```python
from build123d import *

# Parameters (mm, degrees)
ESQUISSE5_W                  = 10
ESQUISSE5_H                  = 23
ESQUISSE5_W_2                = 260
ESQUISSE5_H_2                = 10
ESQUISSE5_W_3                = 9.9238066
BOSS_EXTRU_4_DEPTH           = 81
ENL_V_MAT_EXTRU_2_DEPTH      = 2
ENL_V_MAT_EXTRU_2_DEPTH_BACK = 227


with BuildPart() as part:
    # Esquisse5 → Boss.-Extru.4 (new body)
    with BuildSketch(Plane(origin=(0, 0, 0), x_dir=(1, 0, 0), z_dir=(0, 1, 0))):
        Polygon((0, 32.998552378), (0, 23), (10, 23), (250.0761934, 23), (260, 23), (260, 32.998552378), align=None)
        with Locations((5, 11.5)):
            Rectangle(ESQUISSE5_W, ESQUISSE5_H)
        with Locations((130, -5)):
            Rectangle(ESQUISSE5_W_2, ESQUISSE5_H_2)
        with Locations((255.0380967, 11.5)):
            Rectangle(ESQUISSE5_W_3, ESQUISSE5_H)
    extrude(amount=BOSS_EXTRU_4_DEPTH)

    # Esquisse7 → Enlèv. mat.-Extru.2 (cut, two sides: drawn at the far end of the back side and taken through both)
    with BuildSketch(Plane(origin=(0, 0, -32.998552378), x_dir=(-1, 0, 0), z_dir=(0, 0, -1)).offset(-ENL_V_MAT_EXTRU_2_DEPTH_BACK)):
        Polygon((0, 0), (0, 81), (-39.230090492, 0), align=None)
    extrude(amount=ENL_V_MAT_EXTRU_2_DEPTH + ENL_V_MAT_EXTRU_2_DEPTH_BACK, mode=Mode.SUBTRACT)


solid = part.part
```
Part model, mm, in its own coordinate system. A direction names the side the tool comes from. Give positions to 0.01 mm unless a question says otherwise; leave off trailing zeros. Order: outer loops, then holes, each group sorted by start corner. A loop starts at its lowest first (then second) coordinate and runs counter-clockwise, first axis right, second up. Notation, with made-up numbers: (-16.5, 16.5) - (37.5, 16.5) arc R16 ccw to (37.5, 42.5) - close; hole circle Ø10 at (47, 68.25). An arc over 180 degrees is marked (long way). Use one line per item in the form item = value.
Item 1: Probe probe 1 along Z at (x, y) = (59, 72.5); probe 2 along X at (y, z) = (43, -14); probe 3 along X at (y, z) = (76, -8). List the from-to ranges inside material, lowest first. Write a range as from..to.
Solution:
probe_1 = -33..-23, 0..10
probe_2 = 250.08..260
probe_3 = 2.42..10, 250.08..260
Item 2: Two-plate mould, pull along X, no slides. Class faces 3 (the face through (10, 71, -11)), 4 (the face through (260, 40, -11)), 5 (the face through (148, 0, -26)): released by +X, released by -X, zero draft, split by the parting line, or undercut.
Solution:
face_3 = undercut
face_4 = released by +X
face_5 = zero draft
Item 3: Slice it at C-C on y = 55. Give the cut face in (x, z).
Solution:
outline = (12.59, -33) - (260, -33) - (260, 10) - (12.59, 10) - (12.59, 0) - (250.08, 0) - (250.08, -23) - (12.59, -23) - close
Item 4: Slice it at D-D on y = 73. Give the cut face in (x, z).
Solution:
outline = (3.87, -33) - (260, -33) - (260, 10) - (3.87, 10) - close; hole (10, -23) - (250.08, -23) - (250.08, 0) - (10, 0) - close
Item 5: Which spindle directions (+Z, -Z, +X, -X, +Y, -Y) get a long thin tool onto all of the face, cutting with end or side? Do faces 1 (the face through (14.98, 50.07, 3.13)), 2 (the face through (128, 40, 0)). Say none if no direction does.
Solution:
face_1 = +Z, -Z, -X, -Y
face_2 = +Y, -Y
Item 6: Pin check, flat tips, straight feed: pin 1 Ø5 at (y, z) = (70.5, -23) entering from -X; pin 2 Ø11.5 at (y, z) = (44.5, -15.5) entering from -X; pin 3 Ø8 at (y, z) = (24, -28) entering from -X. Stop position of each tip, or through.
Solution:
pin_1 = 3.87
pin_2 = 250.08
pin_3 = 25.67
Item 7: Slice it at B-B on x = 159. Give the cut face in (y, z).
Solution:
outline = (0, -33) - (81, -33) - (81, -23) - (0, -23) - close; (0, 0) - (81, 0) - (81, 10) - (0, 10) - close
Item 8: Slice it at A-A on z = -7.5. Give the cut face in (x, y).
Solution:
outline = (0, 81) - (10, 60.35) - (10, 81) - close; (250.08, 0) - (260, 0) - (260, 81) - (250.08, 81) - close
